Part model, mm, in its own coordinate system. Face numbers are marked on the shaded views. A direction names the side the tool comes from. Round coordinates to 2 decimals unless told otherwise and drop trailing zeros. Write each loop counter-clockwise with the first axis right and the second up, starting at its lowest first coordinate (ties: lowest second). Pieces come first, ordered by that corner, then holes. Notation, with made-up numbers: (-20, -13) -> (-14, -13) arc R7 ccw to (-14, -8) -> close; hole circle Ø5 at (-26, 37.5). An arc over 180 degrees is marked (long way). Return JSON: item names as keys, results as strings. Group by question number.
(1) Mould opens along Y. For the marked faces 4, 5 and 6 say: +Y half, -Y half, draft (parallel to the pull), parting line (faces both ways), or undercut.
(2) Tool access for the marked faces 1, 2 and 3: list every direction of +Z, -Z, +X, -X, +Y, -Y with a clear straight run to the whole face (end or side of a thin tool).
(3) Saw through at A-A (x = 0). List the corners of the cut face in (y, z) (3 decimals), plus the area to 3 significant figures.
(4) Saw through at B-B (z = -2.5). List the corners of the cut face in (x, y).
(5) Drill centre lines: L1, parallel to Y at x = -4.5, z = 9.5; L2, parallel to Z at x = 0, y = 2.45 (3 decimals); L3, parallel to Y at x = -3.81, z = -10.1. Where is each one in solid material? Low to high. Write a range as from..to.
(6) Drop flat-ended pins along their axis: pin 1 Ø3 at (x, y) = (-3.81, -3.302) entering from -Z; pin 2 Ø0.9 at (x, y) = (3.5, -8) entering from +Z; pin 3 Ø5.5 at (x, y) = (1, -3.5) entering from +Z. Give the stop position or say it passes through.
(7) Saw through at C-C (x = 3.81). List the corners of the cut face in (y, z).
(8) Saw through at D-D (z = 3.75). List the corners of the cut face in (x, y).
from build123d import *

# Parameters (mm, degrees)
SKETCH1_W                 = 14.224
SKETCH1_H                 = 23.622
BOSS_EXTRUDE1_DEPTH       = 3.048
SKETCH2_W                 = 3.175
SKETCH2_H                 = 6.604
MIDDLE_DEPTH              = 14.224
SKETCH3_W                 = 14.224
SKETCH3_H                 = 23.162672358
BOTTOM_DEPTH              = 3.048
SKETCH4_R                 = 3.556
HOLE_FOR_CLEVIS_PIN_DEPTH = 13.7
SKETCH5_R                 = 1.6637
HOLES_FOR_SCREWS_DEPTH    = 24.622


with BuildPart() as part:
    # Sketch1 → Boss-Extrude1 (new body)
    with BuildSketch(Plane(origin=(0, 0, 0), x_dir=(1, 0, 0), z_dir=(0, 1, 0))):
        Rectangle(SKETCH1_W, SKETCH1_H)
    extrude(amount=BOSS_EXTRUDE1_DEPTH)

    # Sketch2 → middle (add)
    with BuildSketch(Plane(origin=(7.112, 0, 0), x_dir=(0, 0, -1), z_dir=(1, 0, 0))):
        with Locations((10.2235, -3.302)):
            Rectangle(SKETCH2_W, SKETCH2_H)
    extrude(amount=-MIDDLE_DEPTH)

    # Sketch3 → bottom (add)
    with BuildSketch(Plane.XZ.offset(6.604)):
        with Locations((0, -0.229663821)):
            Rectangle(SKETCH3_W, SKETCH3_H)
    extrude(amount=BOTTOM_DEPTH)

    # Sketch4 → hole for clevis pin (cut, through all)
    with BuildSketch(Plane(origin=(0, 3.048, 0), x_dir=(1, 0, 0), z_dir=(0, 1, 0))):
        with Locations((0, -4.699)):
            Circle(SKETCH4_R)
    extrude(amount=-HOLE_FOR_CLEVIS_PIN_DEPTH, mode=Mode.SUBTRACT)

    # Sketch5 → holes for screws (cut, through all)
    with BuildSketch(Plane(origin=(0, 0, -11.811), x_dir=(-1, 0, 0), z_dir=(0, 0, -1))):
        with Locations((-3.81, -3.302)):
            Circle(SKETCH5_R)
        with Locations((3.81, -3.302)):
            Circle(SKETCH5_R)
    extrude(amount=-HOLES_FOR_SCREWS_DEPTH, mode=Mode.SUBTRACT)


solid = part.part
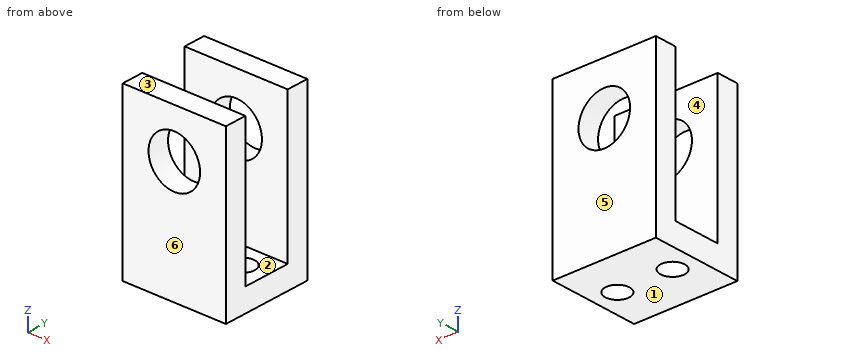
Computed values:
{
 "1": {"face 4": "undercut", "face 5": "+Y half", "face 6": "-Y half"},
 "2": {"face 1": "-Z, +X, -X, +Y, -Y", "face 2": "+Z, +X, -X", "face 3": "+Z, +X, -X, -Y"},
 "3": {"outline": "(-9.652, -11.811) -> (3.048, -11.811) -> (3.048, 1.143) -> (0, 1.143) -> (0, -8.636) -> (-6.604, -8.636) -> (-6.604, 1.143) -> (-9.652, 1.143) -> close; (-9.652, 8.255) -> (-6.604, 8.255) -> (-6.604, 11.352) -> (-9.652, 11.352) -> close; (0, 8.255) -> (3.048, 8.255) -> (3.048, 11.811) -> (0, 11.811) -> close", "area": "120 mm2"},
 "4": {"outline": "(-7.11, -9.65) -> (7.11, -9.65) -> (7.11, -6.6) -> (-7.11, -6.6) -> close; (-7.11, 0) -> (7.11, 0) -> (7.11, 3.05) -> (-7.11, 3.05) -> close"},
 "5": {"L1": "-9.65..-6.6, 0..3.05", "L2": "-11.811..1.143, 8.255..11.811", "L3": "-9.65..-4.97, -1.64..3.05"},
 "6": {"pin 1": "through", "pin 2": "z = 11.35", "pin 3": "z = -8.64"},
 "7": {"outline": "(-9.65, -11.81) -> (-4.97, -11.81) -> (-4.97, -8.64) -> (-6.6, -8.64) -> (-6.6, 11.35) -> (-9.65, 11.35) -> close; (-1.64, -11.81) -> (3.05, -11.81) -> (3.05, 11.81) -> (0, 11.81) -> (0, -8.64) -> (-1.64, -8.64) -> close"},
 "8": {"outline": "(-7.11, -9.65) -> (-3.43, -9.65) -> (-3.43, -6.6) -> (-7.11, -6.6) -> close; (-7.11, 0) -> (-3.43, 0) -> (-3.43, 3.05) -> (-7.11, 3.05) -> close; (3.43, -9.65) -> (7.11, -9.65) -> (7.11, -6.6) -> (3.43, -6.6) -> close; (3.43, 0) -> (7.11, 0) -> (7.11, 3.05) -> (3.43, 3.05) -> close"}
}
